Autodesk Inventor part; units mm, degrees
sketch "スケッチ1" plane through (0, 0, 0) normal (0, 0, 1) x (1, 0, 0)
  circle A0 centre (0, 0) radius 2.875
  dimension "d0" = 5.75
extrude "押し出し1" add sketch "スケッチ1" against normal blind 2.4
sketch "スケッチ2" plane through (0, 0, 0) normal (0, 0, 1) x (1, 0, 0)
  circle A0 centre (0, 0) radius 2.75
  dimension "d3" = 5.5
extrude "押し出し2" add sketch "スケッチ2" along normal blind 1.9
sketch "スケッチ3" plane through (0, 0, 0) normal (0, 0, 1) x (1, 0, 0)
  circle A0 centre (0, 0) radius 4
  circle A1 centre (13.5, 0) radius 3
  line L0 (-5.7629, 0) -> (13.5774, 0)
  line L1 (0.2963, 3.989) -> (13.7222, 2.9918)
  line L2 (13.7222, -2.9918) -> (0.2963, -3.989)
  dimension "d6" = 8
  dimension "d7" = 6
  dimension "d8" = 13.5
extrude "押し出し3" add sketch "スケッチ3" along normal blind 1.4 and the other way blind 0.4
sketch "スケッチ4" plane through (0, 0, 0) normal (0, 0, 1) x (1, 0, 0)
  circle A0 centre (13.5, 0) radius 0.43
  point P0 (0, 0)
  dimension "d13" = 0.86
  dimension "d15" = 13.5
extrude "押し出し4" cut sketch "スケッチ4" along normal through all both and the other way through all
sketch "スケッチ5" plane through (0, 0, 0) normal (0, 0, 1) x (1, 0, 0)
  circle A0 centre (0, 0) radius 1.9
  dimension "d22" = 3.8
extrude "押し出し5" cut sketch "スケッチ5" against normal through all
pattern_linear "矩形状パターン1" count 3 spacing 3 along (-1, 0, 0) of "押し出し4"
properties part number "ASV-15MGSingleHorn01"
Model file for the job. Use its own axes, mm. A direction names the side the tool comes from. Coordinates: 2 decimals unless noted, no trailing zeros. Write each loop counter-clockwise with the first axis right and the second up, starting at its lowest first coordinate (ties: lowest second). Pieces come first, ordered by that corner, then holes. Notation, with made-up numbers: (-18.5, 20) - (36.5, 20) arc R17 ccw to (36.5, 47) - close; hole circle Ø3 at (86.25, 23.5). An arc over 180 degrees is marked (long way). One line per item, written item: value. Start each with the question number.
1. Slice it at D-D (z = 0.65). Write the cut outline in (x, y).
2. Flat gauge pins, fed straight in: pin 1 (2.5 mm diameter, centred on x = 10.5, y = 1, fed in from +Z); pin 2 (1 mm diameter, centred on x = 6, z = 0, fed in from -Y); pin 3 (2.5 mm diameter, centred on x = 9.5, y = -1, fed in from -Z). Where does each tip first touch, or does it go through?
3. Probe line 1 (X direction, y = 0, z = 0.8); line 2 (Y direction, x = 0, z = -0.9) (3 decimals); line 3 (X direction, y = -0.25, z = 0.75). List the from-to ranges inside material, lowest first. Write a range as from..to.
4. Mould opens along X. For faces 1 (the flat face through (6, 0, 1.4)), 2 (the cylindrical face through (7.91, 0.13, 0.51)), 3 (the flat face through (6.9, 3.5, 0.5)), 4 (the cylindrical face through (13.9, -0.16, 0.51)) say: released by +X, released by -X, zero draft, split by the parting line, or undercut.
5. Tool access for faces 5 (the cylindrical face through (-0.596, 2.685, 1.646)), 6 (the flat face through (1, -2, -2.4)), 7 (the cylindrical face through (-1.9, 0.08, -1.18)): list every direction of +Z, -Z, +X, -X, +Y, -Y with a clear straight run to the whole face (end or side of a thin tool).
6. Slice it at A-A (x = 7.5). Write the cut outline in (y, z).
7. Slice it at C-C (x = 0). Write the cut outline in (y, z) (3 decimals), plus the area to 3 significant figures.
8. Slice it at B-B (y = 0). Write the cut outline in (x, z) (3 decimals).
Answers below:
1. outline: (0.3, -3.99) - (13.72, -2.99) arc R3 ccw to (13.72, 2.99) - (0.3, 3.99) arc R4 ccw (long way) to start; hole circle Ø0.86 at (7.5, 0); hole circle Ø0.86 at (10.5, 0); hole circle Ø0.86 at (13.5, 0)
2. pin 1: stops at z = 1.4
2. pin 2: stops at y = -3.6
2. pin 3: stops at z = -0.4
3. line 1: x = -4..7.07, 7.93..10.07, 10.93..13.07, 13.93..16.5
3. line 2: y = -2.875..-1.9, 1.9..2.875
3. line 3: x = -3.99..7.15, 7.85..10.15, 10.85..13.15, 13.85..16.49
4. face 1: zero draft
4. face 2: undercut
4. face 3: released by +X
4. face 4: undercut
5. face 5: +Z
5. face 6: -Z, +X, -X, +Y, -Y
5. face 7: -Z
6. outline: (-3.45, -0.4) - (-0.43, -0.4) - (-0.43, 1.4) - (-3.45, 1.4) - close; (0.43, -0.4) - (3.45, -0.4) - (3.45, 1.4) - (0.43, 1.4) - close
7. outline: (-4, -0.4) - (-2.875, -0.4) - (-2.875, -2.4) - (-1.9, -2.4) - (-1.9, 0) - (1.9, 0) - (1.9, -2.4) - (2.875, -2.4) - (2.875, -0.4) - (4, -0.4) - (4, 1.4) - (2.75, 1.4) - (2.75, 1.9) - (-2.75, 1.9) - (-2.75, 1.4) - (-4, 1.4) - close
7. area: 19.5 mm^2
8. outline: (-4, -0.4) - (-2.875, -0.4) - (-2.875, -2.4) - (-1.9, -2.4) - (-1.9, 0) - (1.9, 0) - (1.9, -2.4) - (2.875, -2.4) - (2.875, -0.4) - (7.07, -0.4) - (7.07, 1.4) - (2.75, 1.4) - (2.75, 1.9) - (-2.75, 1.9) - (-2.75, 1.4) - (-4, 1.4) - close; (7.93, -0.4) - (10.07, -0.4) - (10.07, 1.4) - (7.93, 1.4) - close; (10.93, -0.4) - (13.07, -0.4) - (13.07, 1.4) - (10.93, 1.4) - close; (13.93, -0.4) - (16.5, -0.4) - (16.5, 1.4) - (13.93, 1.4) - close
